Geometry: final body of the model. Coordinates: model frame, mm. Give positions to 0.01 mm unless a question says otherwise; leave off trailing zeros. Loops run counter-clockwise (first coordinate to the right, second up) from the corner with the lowest first, then second, coordinate; pieces in that order, holes last. Notation, with made-up numbers: (49, -3) -> (54, -3) arc R7 cw to (54, 10) -> close; hole circle Ø1 at (69.25, -22.75). An arc over 180 degrees is marked (long way). Answer in a Markdown table with one row per item. Add a question column.
1) Line query: line 1 (Y direction, x = 73, z = 976); line 2 (X direction, y = -52.5, z = 1331); line 3 (Y direction, x = 10.5, z = 174). Output: solid intervals per line, ascending. Write a range as from..to.
2) First-contact query: P1, Ø3, axis at y = -35.5, z = 1122, coming from the -X side. Flat tip, straight axial feed; report the tip coordinate or a pass-through.
3) Section query C-C (y = -26). Return the cut outline in (x, z), plus the area to 3 significant figures.
4) Section query A-A (x = 43.5). Return the cut outline in (y, z), plus the area to 3 significant figures.
5) Section query B-B (z = 1672.5). Return the cut outline in (x, y), plus the area to 3 significant figures.
Autodesk Inventor part; units mm, degrees
ref_plane "Start plane" through (0, 0, 80) normal (0, 0, 1) x (1, 0, 0)
ref_plane "End plane" through (0, 0, 2120) normal (0, 0, 1) x (1, 0, 0)
ref_plane "Work Plane4" through (-3520, 0, 80) normal (0, 0, -1) x (-1, 0, 0)
ref_plane "Start plane" through (0, 0, 80) normal (0, 0, 1) x (1, 0, 0)
ref_plane "End plane" through (0, 0, 2120) normal (0, 0, 1) x (1, 0, 0)
sketch "Sketch" plane through (0, 0, 0) normal (0, 0, 1) x (1, 0, 0)
  line L0 (0, 0) -> (0, 100)
  line L1 (0, 100) -> (80, 100)
  line L2 (80, 100) -> (80, 89)
  line L3 (80, 89) -> (19, 89)
  line L4 (6, 76) -> (6, 0)
  line L5 (6, 0) -> (0, 0) construction
  line L6 (25.6, 100) -> (25.6, 89) construction
  line L7 (80, 89) -> (80, 89) construction
  line L8 (80, 89) -> (25.6, 89) construction
  line L9 (0, 12) -> (0, -30) construction
  line L10 (-1.5, 0) -> (19.5, 0) construction
  line L11 (0, 0) -> (0, -100)
  line L12 (0, -100) -> (80, -100)
  line L13 (80, -100) -> (80, -89)
  line L14 (80, -89) -> (19, -89)
  line L15 (6, -76) -> (6, 0)
  arc A0 (6, -76) -> (19, -89) centre (19, -76) ccw
  arc A1 (19, 89) -> (6, 76) centre (19, 76) ccw
  line L16 (0, 140) -> (0, -140) construction
  line L17 (-17.8, 0) -> (96.3, 0) construction
  point P0 (6, 89)
  point P1 (6, -89)
  point P2 (25.6, -100)
  point P3 (25.6, -89)
  dimension "d0" = 6
  dimension "d1" = 100
  dimension "d2" = 80
  dimension "d3" = 11
  dimension "d5" = 0
  dimension "d23" = 13
  dimension "d24" = 0
  dimension "d29" = 25.6
extrude "Body" add sketch "Sketch" along normal up to surface (2040 mm away) from surface at 80
sketch "Sketch3" plane through (0, 0, 0) normal (0, 0, 1) x (1, 0, 0)
  line L0 (0, 0) -> (10, 0)
ref_plane "Work Plane3" through (0, 0, 0) normal (0, -1, 0) x (1, 0, 0)
sketch "Sketch4" plane through (0, 0, 0) normal (0, -1, 0) x (1, 0, 0)
  line L0 (-2, 80) -> (12, 80)
  line L1 (-2, 2120) -> (12, 2120)
  dimension "d28" = 2040
ref_plane "Work Plane4" through (-3520, 0, 80) normal (0, 0, -1) x (-1, 0, 0)
split "Split1" plane through (-3520, 0, 80) removes the side toward (0, 0, -1)
ref_plane "Work Plane5" through (80, 0, 2120) normal (0, 0, 1) x (1, 0, 0)
split "Split2" plane through (80, 0, 2120) removes the side toward (0, 0, 1)
equation "\"d0\" = G_T"
equation "\"d1\" = 0.5 * G_H"
equation "\"d2\" = G_W"
equation "\"d3\" = G_T1"
equation "\"d23\" = G_IR"
equation "\"d29\" = G_C"
equation "\"d6\" = G_L"
equation "\"G_W\" = 80"
equation "\"G_H\" = 200"
equation "\"G_T\" = 6"
equation "\"G_T1\" = 11"
equation "\"G_NG\" = 0"
equation "\"G_IR\" = 13"
equation "\"G_C\" = 25.6"
equation "\"G_L\" = d28"
equation "\"ex\" = 0"
properties part number "DIN 1026-2 - UPE 200 - 2040" material "Steel, Mild"
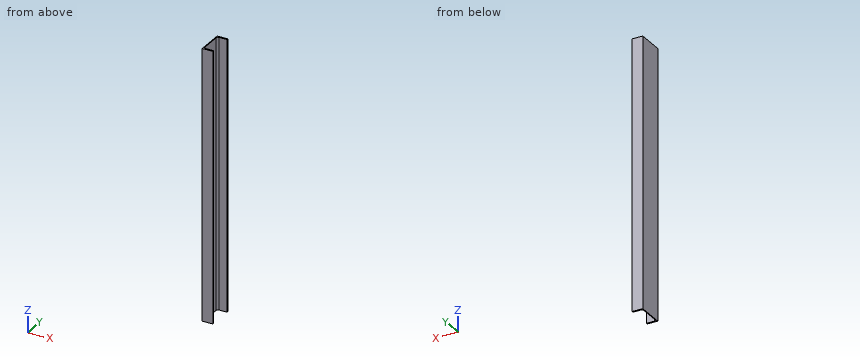
Evaluation:
| question | item | result |
|---|---|---|
| 1 | line 1 | -100..-89, 89..100 |
| 1 | line 2 | 0..6 |
| 1 | line 3 | -100..-85.84, 85.84..100 |
| 2 | P1 | x = 0 |
| 3 | outline | (0, 80) -> (6, 80) -> (6, 2120) -> (0, 2120) -> close |
| 3 | area | 12,200 mm² |
| 4 | outline | (-100, 80) -> (-89, 80) -> (-89, 2120) -> (-100, 2120) -> close; (89, 80) -> (100, 80) -> (100, 2120) -> (89, 2120) -> close |
| 4 | area | 44,900 mm² |
| 5 | outline | (0, -100) -> (80, -100) -> (80, -89) -> (19, -89) arc R13 cw to (6, -76) -> (6, 76) arc R13 cw to (19, 89) -> (80, 89) -> (80, 100) -> (0, 100) -> close |
| 5 | area | 2,900 mm² |
